Part model, mm, in its own coordinate system. Face numbers are marked on the shaded views. A direction names the side the tool comes from. Give positions to 0.01 mm unless a question says otherwise; leave off trailing zeros. Write each loop counter-clockwise with the first axis right and the second up, starting at its lowest first coordinate (ties: lowest second). Pieces come first, ordered by that corner, then holes. Notation, with made-up numbers: M 67.5,-13.5 L 114.5,-13.5 A32 ccw 114.5,16.5 Z; hole C -38.75,46.25 d11. An arc over 180 degrees is marked long. Use a Markdown table: item, result.
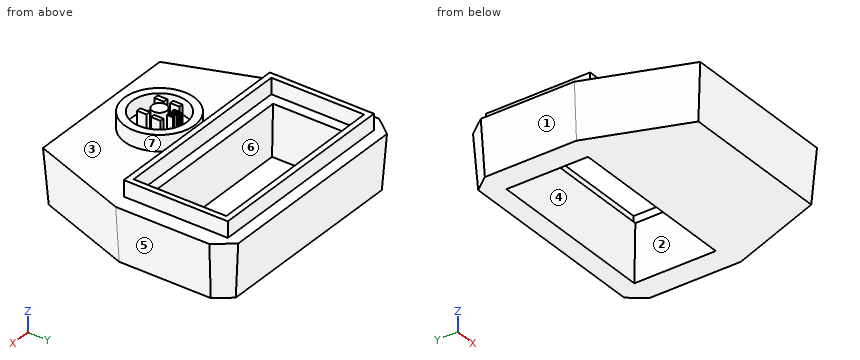
```python
from build123d import *

# Parameters (mm, degrees)
SKETCH1_W           = 154
SKETCH1_H           = 72
BOSS_EXTRUDE1_DEPTH = 48
BOSS_EXTRUDE1_DRAFT = -4
SKETCH2_R           = 31
SKETCH2_R_2         = 24
SKETCH2_W           = 176
SKETCH2_H           = 92
SKETCH2_W_2         = 166
SKETCH2_H_2         = 82
BOSS_EXTRUDE2_DEPTH = 62
SKETCH3_R           = 6.5
SKETCH3_W           = 1.8
SKETCH3_H           = 5.6
SKETCH3_H_2         = 6.4
SKETCH3_W_2         = 3.6
SKETCH3_H_3         = 8.4
SKETCH3_W_3         = 4
BOSS_EXTRUDE3_DEPTH = 65


with BuildPart() as part:
    # Sketch1 → Boss-Extrude1 (with draft: the straight prism first)
    with BuildSketch(Plane.XY):
        Polygon((-88, 90), (-99, 76), (-99, -5), (-68, -90), (68, -90), (99, -5), (99, 76), (88, 90), align=None)
        with Locations((0, 37)):
            Rectangle(SKETCH1_W, SKETCH1_H, mode=Mode.SUBTRACT)
    extrude(amount=BOSS_EXTRUDE1_DEPTH)
    # Boss-Extrude1: the draft: its side faces are tilted about the plane it starts from
    boss_extrude1_sides = [part.faces().sort_by_distance(p)[0] for p in [
        (-93.5, 83, 24),
        (-99, 35.5, 24),
        (-83.5, -47.5, 24),
        (0, -90, 24),
        (83.5, -47.5, 24),
        (99, 35.5, 24),
        (93.5, 83, 24),
        (0, 90, 24),
        (-77, 37, 24),
        (0, 73, 24),
        (77, 37, 24),
        (0, 1, 24),
    ]]
    draft(boss_extrude1_sides, Plane.XY, BOSS_EXTRUDE1_DRAFT)

    # Sketch2 → Boss-Extrude2 (add)
    # profile 1 of 2: a face of its own
    with BuildSketch(Plane.XY):
        with Locations(Location((0, -42, 0), (0, 0, 180))):
            Circle(SKETCH2_R)
        with Locations(Location((0, -42, 0), (0, 0, 180))):
            Circle(SKETCH2_R_2, mode=Mode.SUBTRACT)
    # profile 2 of 2: a face of its own
    with BuildSketch(Plane.XY):
        with Locations((0, 37)):
            Rectangle(SKETCH2_W, SKETCH2_H)
        with Locations((0, 37)):
            Rectangle(SKETCH2_W_2, SKETCH2_H_2, mode=Mode.SUBTRACT)
    extrude(amount=BOSS_EXTRUDE2_DEPTH)

    # Sketch3 → Boss-Extrude3 (add)
    with BuildSketch(Plane.XY):
        with Locations(Location((0, -42, 0), (0, 0, 180))):
            Circle(SKETCH3_R)
        with Locations((-3.5, -29.5)):
            Rectangle(SKETCH3_W, SKETCH3_H)
        with Locations((0, -29)):
            Rectangle(SKETCH3_W, SKETCH3_H_2)
        with Locations((3.5, -29.5)):
            Rectangle(SKETCH3_W, SKETCH3_H)
        with Locations((-11.5, -35.5)):
            Rectangle(SKETCH3_W_2, SKETCH3_H_3)
        with Locations((11.5, -35.5)):
            Rectangle(SKETCH3_W_2, SKETCH3_H_3)
        with Locations((-10.5, -48.5)):
            Rectangle(SKETCH3_W_3, SKETCH3_H_3)
        with Locations((10.5, -48.5)):
            Rectangle(SKETCH3_W_3, SKETCH3_H_3)
    extrude(amount=BOSS_EXTRUDE3_DEPTH)


solid = part.part
```
1. Drop flat-ended pins along their axis: P1, Ø4, axis at x = 11, z = 57.5, coming from the +Y side; P2, Ø10, axis at x = 69.5, y = 26, coming from the +Z side; P3, Ø4, axis at x = -56.5, z = 54.5, coming from the -Y side; P4, Ø24.5, axis at x = 14, y = 20.5, coming from the +Z side. Give the stop position or say it passes through.
Findings below:
| item | result |
|---|---|
| P1 | y = 83 |
| P2 | z = 48 |
| P3 | y = -9 |
| P4 | through |
2. Two-plate mould, pull along X, no slides. Class the marked faces 1, 2, 3 and 4: released by +X, released by -X, zero draft, split by the parting line, or undercut.
Findings below:
| item | result |
|---|---|
| face 1 | released by -X |
| face 2 | undercut |
| face 3 | zero draft |
| face 4 | undercut |
3. Cut at B-B, the plane x = -52.5. Give the cut face in (y, z), then the cut area to 3 significant figures.
Findings below:
| item | result |
|---|---|
| outline | M -93.36,48 L -90,0 L 1,0 L 4.36,48 L -4,48 L -4,62 L -9,62 L -9,48 Z; M 69.64,48 L 73,0 L 90,0 L 93.36,48 L 83,48 L 83,62 L 78,62 L 78,48 Z |
| area | 5,650 mm2 |
4. Cut at C-C, the plane y = 20.5. Give the cut face in (x, z), then the cut area to 3 significant figures.
Findings below:
| item | result |
|---|---|
| outline | M -102.36,48 L -99,0 L -77,0 L -73.64,48 L -83,48 L -83,62 L -88,62 L -88,48 Z; M 73.64,48 L 77,0 L 99,0 L 102.36,48 L 88,48 L 88,62 L 83,62 L 83,48 Z |
| area | 2,570 mm2 |
5. Tool access for the marked faces 5, 6 and 7: list every direction of +Z, -Z, +X, -X, +Y, -Y with a clear straight run to the whole face (end or side of a thin tool).
Findings below:
| item | result |
|---|---|
| face 5 | -Z, +X, +Y, -Y |
| face 6 | -Z |
| face 7 | +Z |
6. Cut at D-D, the plane z = 36.5. Give the cut face in (x, y).
Findings below:
| item | result |
|---|---|
| outline | M -101.55,-5.45 L -69.79,-92.55 L 69.79,-92.55 L 101.55,-5.45 L 101.55,76.88 L 89.24,92.55 L -89.24,92.55 L -101.55,76.88 Z; hole M -74.45,3.55 L 74.45,3.55 L 74.45,70.45 L -74.45,70.45 Z |
7. Drill centre lines: L1, parallel to Y at x = 0, z = 59.25; L2, parallel to X at y = 42, z = 60.5; L3, parallel to Y at x = -16, z = 59.5. Where is each one in solid material? Low to high.
Findings below:
| item | result |
|---|---|
| L1 | -73 to -66, -48.5 to -35.5, -32.2 to -25.8, -18 to -11, -9 to -4, 78 to 83 |
| L2 | -88 to -83, 83 to 88 |
| L3 | -68.55 to -59.89, -24.11 to -15.45, -9 to -4, 78 to 83 |
8. Cut at A-A, the plane z = 52.5. State how many separate pieces and enclosed holes the cut face has, then the cut area to 3 significant figures.
Findings below:
| item | result |
|---|---|
| separate pieces | 10 |
| enclosed holes | 2 |
| area | 4,080 mm2 |
